CAD build for the part. Positions are in the model's coordinates, mm. Face numbers are marked on the shaded views. A direction names the side the tool comes from. Round coordinates to 2 decimals unless told otherwise and drop trailing zeros. Loops run counter-clockwise (first coordinate to the right, second up) from the corner with the lowest first, then second, coordinate; pieces in that order, holes last.
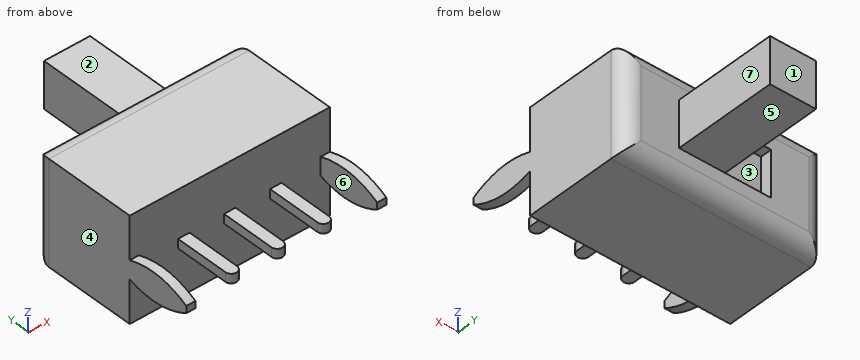
```python
from build123d import *

# Parameters (mm, degrees)
SKETCH1_W           = 8.7
SKETCH1_H           = 4.7
BOSS_EXTRUDE1_DEPTH = 2.25
FILLET1_R           = 0.7
BOSS_EXTRUDE2_DEPTH = 0.4
BOSS_EXTRUDE3_DEPTH = 0.2
SKETCH6_W           = 4
SKETCH6_H           = 2
CUT_EXTRUDE1_DEPTH  = 0.5
SKETCH7_W           = 2
SKETCH7_H           = 2
BOSS_EXTRUDE4_DEPTH = 5


with BuildPart() as part:
    # Sketch1 → Boss-Extrude1 (new, symmetric)
    with BuildSketch(Plane.XY):
        Rectangle(SKETCH1_W, SKETCH1_H)
    extrude(amount=BOSS_EXTRUDE1_DEPTH, both=True)

    # Fillet1
    fillet1_edges = [part.edges().sort_by_distance(p)[0] for p in [
        (0, 2.35, -2.25),
        (0, 2.35, 2.25),
        (-4.35, 2.35, 0),
        (4.35, 2.35, 0),
    ]]
    fillet(fillet1_edges, radius=FILLET1_R)

    # Sketch3 → Boss-Extrude2 (add)
    with BuildSketch(Plane.ZY.offset(4.35)):
        with BuildLine():
            Line((-0.15, -5.15), (0.15, -5.15))
            add(Edge.make_bspline(
                [(0.4, -2.35), (0.9, -3.820089362), (0.15, -5.15)],
                knots=[0, 0, 0, 1, 1, 1], degree=2))
            Line((0.4, -2.35), (-0.4, -2.35))
            add(Edge.make_bspline(
                [(-0.4, -2.35), (-0.9, -3.820089362), (-0.15, -5.15)],
                knots=[0, 0, 0, 1, 1, 1], degree=2))
        make_face()
    boss_extrude2 = extrude(amount=-BOSS_EXTRUDE2_DEPTH)

    # Mirror1: Boss-Extrude2 across plane
    add(boss_extrude2.mirror(Plane(origin=(0, 0, 0), x_dir=(0, 0, 1), z_dir=(1, 0, 0))))

    # Sketch5 → Boss-Extrude3 (add, symmetric)
    with BuildSketch(Plane.XY):
        with BuildLine():
            Line((-0.25, -2.35), (0.25, -2.35))
            Line((0.25, -2.35), (0.25, -4.7))
            ThreePointArc((0.25, -4.7), (0, -4.95), (-0.25, -4.7))
            Line((-0.25, -4.7), (-0.25, -2.35))
        make_face()
        with BuildLine():
            Line((1.75, -2.35), (2.25, -2.35))
            Line((2.25, -2.35), (2.25, -4.7))
            ThreePointArc((2.25, -4.7), (2, -4.95), (1.75, -4.7))
            Line((1.75, -4.7), (1.75, -2.35))
        make_face()
        with BuildLine():
            Line((-1.75, -2.35), (-1.75, -4.7))
            ThreePointArc((-1.75, -4.7), (-2, -4.95), (-2.25, -4.7))
            Line((-2.25, -4.7), (-2.25, -2.35))
            Line((-2.25, -2.35), (-1.75, -2.35))
        make_face()
    extrude(amount=BOSS_EXTRUDE3_DEPTH, both=True)

    # Sketch6 → Cut-Extrude1 (cut)
    with BuildSketch(Plane(origin=(0, 2.35, 0), x_dir=(1, 0, 0), z_dir=(0, 1, 0))):
        Rectangle(SKETCH6_W, SKETCH6_H)
    extrude(amount=-CUT_EXTRUDE1_DEPTH, mode=Mode.SUBTRACT)

    # Sketch7 → Boss-Extrude4 (add)
    with BuildSketch(Plane(origin=(0, 1.85, 0), x_dir=(1, 0, 0), z_dir=(0, 1, 0))):
        with Locations((1, 0)):
            Rectangle(SKETCH7_W, SKETCH7_H)
    extrude(amount=BOSS_EXTRUDE4_DEPTH)


solid = part.part
```
Item 1: Two-plate mould, pull along X, no slides. Class the marked faces 4, 5, 6 and 7: released by +X, released by -X, zero draft, split by the parting line, or undercut.
Answers follow:
face 4: released by -X
face 5: zero draft
face 6: undercut
face 7: released by +X
Item 2: Cut at B-B, the plane x = 2.5. Give the cut face in (y, z), plus the area to 3 significant figures.
Answers follow:
outline: (-2.35, -2.25) - (1.65, -2.25) arc R0.7 ccw to (2.35, -1.55) - (2.35, 1.55) arc R0.7 ccw to (1.65, 2.25) - (-2.35, 2.25) - close
area: 20.9 mm2
Item 3: 3-axis set-ups, long thin cutter, end or side, ignore diameter. For the marked faces 1, 2 and 3: which of +Z, -Z, +X, -X, +Y, -Y reach the whole face in a straight line?
Answers follow:
face 1: +Z, -Z, +X, -X, +Y
face 2: +Z, +X, -X, +Y
face 3: +Y
Item 4: Cut at D-D, the plane x = 0.75. Give the cut face in (y, z), plus the area to 3 significant figures.
Answers follow:
outline: (-2.35, -2.25) - (1.65, -2.25) arc R0.7 ccw to (2.35, -1.55) - (2.35, -1) - (6.85, -1) - (6.85, 1) - (2.35, 1) - (2.35, 1.55) arc R0.7 ccw to (1.65, 2.25) - (-2.35, 2.25) - close
area: 29.9 mm2
Item 5: Cut at C-C, the plane y = 6.25. Give the cut face in (x, z).
Answers follow:
outline: (0, -1) - (2, -1) - (2, 1) - (0, 1) - close
Item 6: Flat gauge pins, fed straight in: P1, Ø0.6, axis at x = 1, y = 4, coming from the -Z side; P2, Ø0.6, axis at x = -1.5, z = 0.5, coming from the +Y side; P3, Ø0.6, axis at x = 2, y = -4, coming from the +Z side. Where does each tip first touch, or does it go through?
Answers follow:
P1: stops at z = -1
P2: stops at y = 1.85
P3: stops at z = 0.2
Item 7: Cut at A-A, the plane z = -0.8. Give the cut face in (x, y).
Answers follow:
outline: (-4.35, -2.35) - (4.35, -2.35) - (4.35, 1.65) arc R0.7 ccw to (3.65, 2.35) - (2, 2.35) - (2, 6.85) - (0, 6.85) - (0, 1.85) - (-2, 1.85) - (-2, 2.35) - (-3.65, 2.35) arc R0.7 ccw to (-4.35, 1.65) - close
Item 8: Probe line 1 (Y direction, x = 3.25, z = 1.4); line 2 (Y direction, x = -1.25, z = -0.2); line 3 (Z direction, x = -3.5, y = 1.75). List the from-to ranges inside material, lowest first.
Answers follow:
line 1: y = -2.35 to 2.35
line 2: y = -2.35 to 1.85
line 3: z = -2.24 to 2.24
